from build123d import *

# Parameters (mm, degrees)
SKETCH1_W               = 101.6
SKETCH1_H               = 31.75
SKETCH1_R               = 3.175
BOSS_EXTRUDE1_DEPTH     = 12.7
F_1_4_20_TAPPED_HOLE1_D = 5.1054


with BuildPart() as part:
    # Sketch1 → Boss-Extrude1 (new body)
    with BuildSketch(Plane(origin=(0, 0, 0), x_dir=(1, 0, 0), z_dir=(0, 1, 0))):
        with Locations((19.385978836, 15.875)):
            Rectangle(SKETCH1_W, SKETCH1_H)
        with Locations((-18.714021164, 15.875)):
            Circle(SKETCH1_R, mode=Mode.SUBTRACT)
        with Locations((57.485978836, 15.875)):
            Circle(SKETCH1_R, mode=Mode.SUBTRACT)
        with Locations((-2.204021164, 15.875)):
            Circle(SKETCH1_R, mode=Mode.SUBTRACT)
        with Locations((40.975978836, 15.875)):
            Circle(SKETCH1_R, mode=Mode.SUBTRACT)
    extrude(amount=BOSS_EXTRUDE1_DEPTH)

    # 1/4-20 Tapped Hole1 (through all)
    with Locations(Plane(origin=(19.385978836, 6.35, 0), x_dir=(1, 0, 0), z_dir=(0, 0, 1))):
        with Locations((0, 0)):
            Hole(F_1_4_20_TAPPED_HOLE1_D / 2)


solid = part.part
Could you check a few things on this model? Use its own coordinates, in mm. Give positions to 0.01 mm unless a question says otherwise; leave off trailing zeros. Write each loop counter-clockwise with the first axis right and the second up, starting at its lowest first coordinate (ties: lowest second). Pieces come first, ordered by that corner, then holes. Notation, with made-up numbers: (-7, -1.75) - (23, -1.75) arc R7 cw to (23, 6.25) - close; hole circle Ø8 at (-10, 80.25). An arc over 180 degrees is marked (long way). Use CSV: the item, a comma, the result in double quotes. Start each with the question number.
Item 1: I want a section at C-C, the plane x = -18. Please give me the cut outline in (y, z).
Item 2: I want a section at A-A, the plane y = 5.25. Please give me the cut outline in (x, z) (3 decimals).
Item 3: If we mould it in two halves opening along Y, with no side actions, what happens to faces 1 (the face through (21.936, 6.462, -16.097)), 2 (the face through (19, 12.7, -16)), 3 (the face through (-31.414, 6, -16))? For each: pulls with the +Y half, pulls with the -Y half, needs draft (parallel to the pull), parting line crosses it, or undercut.
Item 4: I'm going to push a flat-ended pin straight in: pin 1 (4 mm diameter, centred on x = -4, z = -19, fed in from -Y). Where does the tip first touch, or does it pass through?
Item 5: If I drill on line 1 along X through (y, z) = (2.5, -17); line 2 along X through (y, z) = (3.75, -13.5); line 3 along X through (y, z) = (4, -11), over which ranges is the centre line in solid material (lowest first)?
Item 6: I want a section at B-B, the plane z = -14. Please give me the cut outline in (x, y), then the cut area to 3 significant figures.
Item 7: I want a section at D-D, the plane z = -3. Please give me the cut outline in (x, y), then the cut area to 3 significant figures.
Findings:
1,outline,"(0, -31.75) - (12.7, -31.75) - (12.7, -18.97) - (0, -18.97) - close; (0, -12.78) - (12.7, -12.78) - (12.7, 0) - (0, 0) - close"
2,outline,"(-31.414, -31.75) - (17.082, -31.75) - (17.082, 0) - (-31.414, 0) - close; (21.69, -31.75) - (70.186, -31.75) - (70.186, 0) - (21.69, 0) - close; hole circle Ø6.35 at (-18.714, -15.875); hole circle Ø6.35 at (-2.204, -15.875); hole circle Ø6.35 at (40.976, -15.875); hole circle Ø6.35 at (57.486, -15.875)"
3,face 1,"undercut"
3,face 2,"pulls with the +Y half"
3,face 3,"needs draft"
4,pin 1,"stops at y = 0"
5,line 1,"x = -31.41 to -21.68, -15.75 to -5.17, 0.76 to 38.01, 43.94 to 54.52, 60.45 to 70.19"
5,line 2,"x = -31.41 to -20.82, -16.61 to -4.31, -0.1 to 38.87, 43.08 to 55.38, 59.59 to 70.19"
5,line 3,"x = -31.41 to 18.39, 20.38 to 70.19"
6,outline,"(-31.41, 0) - (-21.28, 0) - (-21.28, 12.7) - (-31.41, 12.7) - close; (-16.15, 0) - (-4.77, 0) - (-4.77, 12.7) - (-16.15, 12.7) - close; (0.36, 0) - (38.41, 0) - (38.41, 12.7) - (0.36, 12.7) - close; (43.54, 0) - (54.92, 0) - (54.92, 12.7) - (43.54, 12.7) - close; (60.05, 0) - (70.19, 0) - (70.19, 12.7) - (60.05, 12.7) - close; hole circle Ø5.11 at (19.39, 6.35)"
6,area,"1,010 mm2"
7,outline,"(-31.41, 0) - (70.19, 0) - (70.19, 12.7) - (-31.41, 12.7) - close; hole circle Ø5.11 at (19.39, 6.35)"
7,area,"1,270 mm2"
